Input: part model. Units: mm. Frame: model coordinates. Coordinates: 2 decimals unless noted, no trailing zeros. Loops run counter-clockwise (first coordinate to the right, second up) from the corner with the lowest first, then second, coordinate; pieces in that order, holes last. Notation, with made-up numbers: (-7, 76) - (49, 76) arc R11 ccw to (49, 96) - close; hole circle Ø8 at (57.5, 57.25). An arc over 180 degrees is marked (long way). Use a Markdown table: item, result. Add a question column.
1. Contact query for flat-ended pins moving along their axis: P1, Ø1.5, axis at x = 59.5, y = 2.5, coming from the +Z side; P2, Ø2, axis at x = -61.5, y = 5, coming from the +Z side; P3, Ø1.5, axis at y = 2.5, z = 56, coming from the -X side. Output: stop coordinate, or through.
2. Section query A-A on z = -82. Return the cut outline in (x, y), then the cut area to 3 significant figures.
3. Ray query, L1, parallel to X at y = 3.5, z = -65 (3 decimals); L2, parallel to X at y = 3.5, z = -62.5; L3, parallel to Z at x = -70, y = 3. Return the intervals inside material, ascending. Write a range as [from, to].
4. Section query C-C on y = 4. State how many separate pieces and enclosed holes the cut face has, then the cut area to 3 significant figures.
5. Section query D-D on z = -56.5. Return the cut outline in (x, y), then the cut area to 3 significant figures.
6. Section query B-B on z = 65. Return the cut outline in (x, y) (3 decimals), then the cut area to 3 significant figures.
```python
from build123d import *

# Parameters (mm, degrees)
ESQUISSE1_R             = 5.7
ESQUISSE1_R_2           = 3.925
BOSS_EXTRU_1_DEPTH      = 6.35
ESQUISSE4_R             = 2.5
ENL_V_MAT_EXTRU_1_DEPTH = 6.35
ESQUISSE5_R             = 4
ENL_V_MAT_EXTRU_2_DEPTH = 135.686014493
ESQUISSE6_R             = 5.7
ENL_V_MAT_EXTRU_3_DEPTH = 135.686014493


with BuildPart() as part:
    # Esquisse1 → Boss.-Extru.1 (new body)
    with BuildSketch(Plane(origin=(0, 0, 0), x_dir=(1, 0, 0), z_dir=(0, 1, 0))):
        with BuildLine():
            Line((-96.654639651, 52.506938663), (-21.654639651, -77.493061337))
            ThreePointArc((-21.654639651, -77.493061337), (0, -90), (21.654639651, -77.493061337))
            Line((21.654639651, -77.493061337), (96.654639651, 52.506938663))
            ThreePointArc((96.654639651, 52.506938663), (96.648631983, 77.50346885), (75, 90))
            Line((75, 90), (-75, 90))
            ThreePointArc((-75, 90), (-96.648631983, 77.50346885), (-96.654639651, 52.506938663))
        make_face()
        with Locations(Location((0, 65, 0), (0, 0, 270))):
            Circle(ESQUISSE1_R, mode=Mode.SUBTRACT)
        with Locations(Location((-75, 65, 0), (0, 0, 270))):
            Circle(ESQUISSE1_R_2, mode=Mode.SUBTRACT)
        with Locations(Location((75, 65, 0), (0, 0, 270))):
            Circle(ESQUISSE1_R_2, mode=Mode.SUBTRACT)
        with Locations(Location((0, -65, 0), (0, 0, 270))):
            Circle(ESQUISSE1_R_2, mode=Mode.SUBTRACT)
    extrude(amount=BOSS_EXTRU_1_DEPTH)

    # Esquisse4 → Enlèv. mat.-Extru.1 (cut)
    with BuildSketch(Plane.XZ):
        with Locations(Location((-75, -82, 0), (0, 0, 90))):
            Circle(ESQUISSE4_R)
        with Locations(Location((-89.722431864, -56.5, 0), (0, 0, 90))):
            Circle(ESQUISSE4_R)
        with Locations(Location((-60.277568136, -56.5, 0), (0, 0, 90))):
            Circle(ESQUISSE4_R)
        with Locations(Location((60.27903399, -56.499154304, 0), (0, 0, 90))):
            Circle(ESQUISSE4_R)
        with Locations(Location((75.001465855, -81.999154304, 0), (0, 0, 90))):
            Circle(ESQUISSE4_R)
        with Locations(Location((89.723897719, -56.499154304, 0), (0, 0, 90))):
            Circle(ESQUISSE4_R)
        with Locations(Location((14.722431864, 56.5, 0), (0, 0, 90))):
            Circle(ESQUISSE4_R)
        with Locations(Location((0, 82, 0), (0, 0, 90))):
            Circle(ESQUISSE4_R)
        with Locations(Location((-14.722431864, 56.5, 0), (0, 0, 90))):
            Circle(ESQUISSE4_R)
    extrude(amount=-ENL_V_MAT_EXTRU_1_DEPTH, mode=Mode.SUBTRACT)

    # Esquisse5 → Enlèv. mat.-Extru.2 (cut, through all)
    with BuildSketch(Plane(origin=(0, 6.35, 0), x_dir=(1, 0, 0), z_dir=(0, 1, 0))):
        with Locations(Location((0.000849353, 10.324999995, 0), (0, 0, 270))):
            Circle(ESQUISSE5_R)
    extrude(amount=-ENL_V_MAT_EXTRU_2_DEPTH, mode=Mode.SUBTRACT)

    # Esquisse6 → Enlèv. mat.-Extru.3 (cut, through all)
    with BuildSketch(Plane(origin=(0, 6.35, 0), x_dir=(1, 0, 0), z_dir=(0, 1, 0))):
        with Locations(Location((0, -21, 0), (0, 0, 270))):
            Circle(ESQUISSE6_R)
    extrude(amount=-ENL_V_MAT_EXTRU_3_DEPTH, mode=Mode.SUBTRACT)


solid = part.part
```
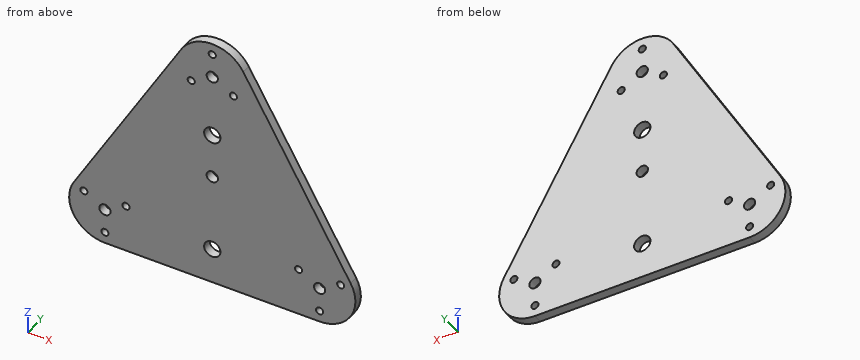
Resolved:
| question | item | result |
|---|---|---|
| 1 | P1 | z = 13.19 |
| 1 | P2 | z = 10.16 |
| 1 | P3 | x = -34.49 |
| 2 | outline | (-93.33, 0) - (-77.5, 0) - (-77.5, 6.35) - (-93.33, 6.35) - close; (-72.5, 0) - (72.5, 0) - (72.5, 6.35) - (-72.5, 6.35) - close; (77.5, 0) - (93.33, 0) - (93.33, 6.35) - (77.5, 6.35) - close |
| 2 | area | 1,120 mm² |
| 3 | L1 | [-100, -78.925], [-71.075, -5.7], [5.7, 71.075], [78.925, 100] |
| 3 | L2 | [-99.87, -78.03], [-71.97, -5.12], [5.12, 71.97], [78.03, 99.87] |
| 3 | L3 | [-90, -6.31] |
| 4 | separate pieces | 1 |
| 4 | enclosed holes | 15 |
| 4 | area | 22,400 mm² |
| 5 | outline | (-98.51, 0) - (-92.22, 0) - (-92.22, 6.35) - (-98.51, 6.35) - close; (-87.22, 0) - (-62.78, 0) - (-62.78, 6.35) - (-87.22, 6.35) - close; (-57.78, 0) - (57.78, 0) - (57.78, 6.35) - (-57.78, 6.35) - close; (62.78, 0) - (87.22, 0) - (87.22, 6.35) - (62.78, 6.35) - close; (92.22, 0) - (98.51, 0) - (98.51, 6.35) - (92.22, 6.35) - close |
| 5 | area | 1,120 mm² |
| 6 | outline | (-28.862, 0) - (-3.925, 0) - (-3.925, 6.35) - (-28.862, 6.35) - close; (3.925, 0) - (28.862, 0) - (28.862, 6.35) - (3.925, 6.35) - close |
| 6 | area | 317 mm² |
